```python
from build123d import *

# Parameters (mm, degrees)
SKETCH2_W           = 36.5
SKETCH2_H           = 27.5
SKETCH2_R           = 11.5
SKETCH2_R_2         = 1
BOSS_EXTRUDE1_DEPTH = 1
SKETCH4_R           = 1
BOSS_EXTRUDE2_DEPTH = 3
SKETCH5_W           = 1.5
SKETCH5_H           = 27.5
BOSS_EXTRUDE3_DEPTH = 12
SKETCH6_W           = 9
SKETCH6_H           = 21.5
CUT_EXTRUDE1_DEPTH  = 1.5
BOSS_EXTRUDE4_DEPTH = 16


with BuildPart() as part:
    # Sketch2 → Boss-Extrude1 (new body)
    with BuildSketch(Plane.XY):
        Rectangle(SKETCH2_W, SKETCH2_H)
        Circle(SKETCH2_R, mode=Mode.SUBTRACT)
        with Locations((-14.75, 0)):
            Circle(SKETCH2_R_2, mode=Mode.SUBTRACT)
        with Locations((14.75, 0)):
            Circle(SKETCH2_R_2, mode=Mode.SUBTRACT)
    extrude(amount=-BOSS_EXTRUDE1_DEPTH)

    # Sketch4 → Boss-Extrude2 (add)
    with BuildSketch(Plane(origin=(0, 0, -1), x_dir=(-1, 0, 0), z_dir=(0, 0, -1))):
        with BuildLine():
            Line((-16.75, 13.75), (-16.75, 4))
            ThreePointArc((-16.75, 4), (-16.164213562, 2.585786438), (-14.75, 2))
            ThreePointArc((-14.75, 2), (-12.75, 0), (-14.75, -2))
            ThreePointArc((-14.75, -2), (-16.164213562, -2.585786438), (-16.75, -4))
            Line((-16.75, -4), (-16.75, -13.75))
            Line((-16.75, -13.75), (-18.25, -13.75))
            Line((-18.25, -13.75), (-18.25, 13.75))
            Line((-18.25, 13.75), (-16.75, 13.75))
        make_face()
        with Locations(Location((-14.75, 0, 0), (0, 0, 180))):
            Circle(SKETCH4_R, mode=Mode.SUBTRACT)
    boss_extrude2 = extrude(amount=BOSS_EXTRUDE2_DEPTH)

    # Sketch5 → Boss-Extrude3 (add)
    with BuildSketch(Plane(origin=(0, 0, -4), x_dir=(-1, 0, 0), z_dir=(0, 0, -1))):
        with Locations((-17.5, 0)):
            Rectangle(SKETCH5_W, SKETCH5_H)
    boss_extrude3 = extrude(amount=BOSS_EXTRUDE3_DEPTH)

    # Sketch6 → Cut-Extrude1 (cut)
    with BuildSketch(Plane(origin=(18.25, 0, 0), x_dir=(0, 0, -1), z_dir=(1, 0, 0))):
        with Locations((8.5, 0)):
            Rectangle(SKETCH6_W, SKETCH6_H)
    cut_extrude1 = extrude(amount=-CUT_EXTRUDE1_DEPTH, mode=Mode.SUBTRACT)

    # Sketch7 → Boss-Extrude4 (add)
    with BuildSketch(Plane(origin=(0, 0, -16), x_dir=(-1, 0, 0), z_dir=(0, 0, -1))):
        Polygon((-18.25, 12.75), (-19.75, 13.616025404), (-19.75, 10.883974596), (-18.25, 11.75), align=None)
        Polygon((-19.75, -10.883974596), (-18.25, -11.75), (-18.25, -12.75), (-19.75, -13.616025404), align=None)
    boss_extrude4 = extrude(amount=-BOSS_EXTRUDE4_DEPTH)

    # Mirror1: Boss-Extrude2, Boss-Extrude3, Cut-Extrude1, Boss-Extrude4 across plane
    add(boss_extrude2.mirror(Plane(origin=(0, 0, 0), x_dir=(0, 0, 1), z_dir=(1, 0, 0))))
    add(boss_extrude3.mirror(Plane(origin=(0, 0, 0), x_dir=(0, 0, 1), z_dir=(1, 0, 0))))
    add(cut_extrude1.mirror(Plane(origin=(0, 0, 0), x_dir=(0, 0, 1), z_dir=(1, 0, 0))), mode=Mode.SUBTRACT)
    add(boss_extrude4.mirror(Plane(origin=(0, 0, 0), x_dir=(0, 0, 1), z_dir=(1, 0, 0))))


solid = part.part
```
Here's how the part is built. I have some questions about the finished solid (model axes, mm). A direction names the side the tool comes from. Give positions to 0.01 mm unless a question says otherwise; leave off trailing zeros. Order: outer loops, then holes, each group sorted by start corner. A loop starts at its lowest first (then second) coordinate and runs counter-clockwise, first axis right, second up. Notation, with made-up numbers: (39.25, 13.5) - (73.25, 13.5) arc R26 cw to (73.25, 37.5) - close; hole circle Ø11 at (22.25, 77). An arc over 180 degrees is marked (long way). Answer as a JSON object with one key per item and string values. Group by question number.
Item 1: Please list where these lines run through material, in increasing order: probe 1 along X at (y, z) = (9.5, -2.5); probe 2 along Y at (x, z) = (14.75, -1.9); probe 3 along Y at (x, z) = (14.75, -0.3).
Item 2: If we section it at B-B on x = 0: Please give me the cut outline in (y, z), and give its area (3 significant figures).
Item 3: Which directions (+Z, -Z, +X, -X, +Y, -Y) give clear straight access to the entire face, cutting with the end or side of a thin tool? Please do faces 4 (the flat face through (-18, 0, -16)), 5 (the flat face through (18, 10.75, -8)), 6 (the flat face through (-16.75, -0.2, -13.4)).
Item 4: If we mould it in two halves opening along X, with no side actions, what happens to faces 1 (the flat face through (19.75, 12, -8)), 2 (the flat face through (19.01, 11.31, -8.11)), 3 (the flat face through (-17, 0, -4))? For each: pulls with the +X half, pulls with the -X half, needs draft (parallel to the pull), parting line crosses it, or undercut.
Item 5: If we section it at A-A on z = -2.25: Give the number of separate pieces and of enclosed holes in the cut face, and give its area (3 significant figures).
Item 6: If we section it at D-D on y = -0.5: Please give me the cut outline in (x, z), and give its area (3 significant figures).
Item 7: For P1, Ø8, axis at x = 12.5, y = -0.5, coming from the -Z side; P2, Ø10, axis at x = 10.5, y = 6, coming from the -Z side; P3, Ø5, axis at y = 3.5, z = -11, coming from the +X side, each with a flat end and sliding along its axis, tell me the tip position at first contact or that it passes through.
Result set:
{
 "1": {"probe 1": "-18.25 to -16.75, 16.75 to 18.25", "probe 2": "-2 to -1, 1 to 2", "probe 3": "-13.75 to -1, 1 to 13.75"},
 "2": {"outline": "(-13.75, -1) - (-11.5, -1) - (-11.5, 0) - (-13.75, 0) - close; (11.5, -1) - (13.75, -1) - (13.75, 0) - (11.5, 0) - close", "area": "4.50 mm²"},
 "3": {"face 4": "-Z, +X, -X, +Y, -Y", "face 5": "+X, -X", "face 6": "-Z"},
 "4": {"face 1": "pulls with the +X half", "face 2": "undercut", "face 3": "needs draft"},
 "5": {"separate pieces": "2", "enclosed holes": "2", "area": "119 mm²"},
 "6": {"outline": "(-18.25, -16) - (-16.75, -16) - (-16.75, -13) - (-18.25, -13) - close; (-18.25, -4) - (-15.62, -4) - (-15.62, 0) - (-18.25, 0) - close; (-13.88, -4) - (-12.81, -4) - (-12.81, -1) - (-11.49, -1) - (-11.49, 0) - (-13.88, 0) - close; (11.49, -1) - (12.81, -1) - (12.81, -4) - (13.88, -4) - (13.88, 0) - (11.49, 0) - close; (15.62, -4) - (18.25, -4) - (18.25, 0) - (15.62, 0) - close; (16.75, -16) - (18.25, -16) - (18.25, -13) - (16.75, -13) - close", "area": "41.3 mm²"},
 "7": {"P1": "z = -4", "P2": "z = -1", "P3": "x = 18.25"}
}
